```python
from build123d import *

# Parameters (mm, degrees)
CROQUIS1_W              = 91.2
CROQUIS1_H              = 54
SALIENTE_EXTRUIR1_DEPTH = 2
CROQUIS2_R              = 2.5
SALIENTE_EXTRUIR2_DEPTH = 4
CROQUIS3_R              = 1.5
CORTAR_EXTRUIR1_DEPTH   = 4
CROQUIS4_W              = 91.2
CROQUIS4_H              = 54
CROQUIS4_W_2            = 85.2
CROQUIS4_H_2            = 48
SALIENTE_EXTRUIR3_DEPTH = 24
CROQUIS7_W              = 87.2
CROQUIS7_H              = 50
CORTAR_EXTRUIR2_DEPTH   = 14
CROQUIS9_W              = 12
CROQUIS9_H              = 25
CORTAR_EXTRUIR3_DEPTH   = 8


with BuildPart() as part:
    # Croquis1 → Saliente-Extruir1 (new body)
    with BuildSketch(Plane(origin=(0, 0, 0), x_dir=(1, 0, 0), z_dir=(0, 1, 0))):
        with Locations((3, 0)):
            Rectangle(CROQUIS1_W, CROQUIS1_H)
    extrude(amount=SALIENTE_EXTRUIR1_DEPTH)

    # Croquis2 → Saliente-Extruir2 (add)
    with BuildSketch(Plane(origin=(0, 2, 0), x_dir=(1, 0, 0), z_dir=(0, 1, 0))):
        with Locations(Location((-9.6, -19, 0), (0, 0, 90))):
            Circle(CROQUIS2_R)
        with Locations(Location((-9.6, 19, 0), (0, 0, 90))):
            Circle(CROQUIS2_R)
        with Locations(Location((33.4, 19, 0), (0, 0, 90))):
            Circle(CROQUIS2_R)
        with Locations(Location((33.4, -19, 0), (0, 0, 90))):
            Circle(CROQUIS2_R)
    extrude(amount=SALIENTE_EXTRUIR2_DEPTH)

    # Croquis3 → Cortar-Extruir1 (cut)
    with BuildSketch(Plane(origin=(0, 6, 0), x_dir=(1, 0, 0), z_dir=(0, 1, 0))):
        with Locations(Location((-9.6, -19, 0), (0, 0, 270))):
            Circle(CROQUIS3_R)
        with Locations(Location((33.4, -19, 0), (0, 0, 270))):
            Circle(CROQUIS3_R)
        with Locations(Location((33.4, 19, 0), (0, 0, 270))):
            Circle(CROQUIS3_R)
        with Locations(Location((-9.6, 19, 0), (0, 0, 270))):
            Circle(CROQUIS3_R)
    extrude(amount=-CORTAR_EXTRUIR1_DEPTH, mode=Mode.SUBTRACT)

    # Croquis4 → Saliente-Extruir3 (add)
    with BuildSketch(Plane(origin=(0, 2, 0), x_dir=(1, 0, 0), z_dir=(0, 1, 0))):
        with Locations((3, 0)):
            Rectangle(CROQUIS4_W, CROQUIS4_H)
        with Locations((3, 0)):
            Rectangle(CROQUIS4_W_2, CROQUIS4_H_2, mode=Mode.SUBTRACT)
    extrude(amount=SALIENTE_EXTRUIR3_DEPTH)

    # Croquis7 → Cortar-Extruir2 (cut)
    with BuildSketch(Plane(origin=(0, 26, 0), x_dir=(1, 0, 0), z_dir=(0, 1, 0))):
        with Locations((3, 0)):
            Rectangle(CROQUIS7_W, CROQUIS7_H)
    extrude(amount=-CORTAR_EXTRUIR2_DEPTH, mode=Mode.SUBTRACT)

    # Croquis9 → Cortar-Extruir3 (cut)
    with BuildSketch(Plane(origin=(0, 26, 0), x_dir=(1, 0, 0), z_dir=(0, 1, 0))):
        with Locations((-25, -23)):
            Rectangle(CROQUIS9_W, CROQUIS9_H)
    extrude(amount=-CORTAR_EXTRUIR3_DEPTH, mode=Mode.SUBTRACT)


solid = part.part
```
The listing builds one solid part. Answer for the finished solid, in the listing's coordinates (mm). A direction names the side the tool comes from. Give positions to 0.01 mm unless a question says otherwise; leave off trailing zeros. Order: outer loops, then holes, each group sorted by start corner. A loop starts at its lowest first (then second) coordinate and runs counter-clockwise, first axis right, second up. Notation, with made-up numbers: M 24.5,53 L 52.5,53 A26 cw 52.5,70 Z; hole C 76,4.5 d6. An arc over 180 degrees is marked long. Put each result on its own line as item: value. Start each with the question number.
Item 1: Find the intervals of material crossed by line 1 along X through (y, z) = (3.45, 19); line 2 along X through (y, z) = (2.5, -17); line 3 along X through (y, z) = (10.75, 20.5), in increasing order.
Item 2: The part is cut by section C-C, the plane z = -19. Determine the outline of the cut face in (x, y).
Item 3: Which of the six approach directions +Z, -Z, +X, -X, +Y, -Y give full straight-line access (tool end or side, diameter ignored) to faces 1 (the face through (2, 13, -27)), 2 (the face through (32.5, 4, -20.2)), 3 (the face through (-25, 18, 26))?
Item 4: The part is cut by section B-B, the plane x = -24. Determine the outline of the cut face in (y, z).
Item 5: The part is cut by section D-D, the plane y = 19.5. Determine the outline of the cut face in (x, z), and give its area (3 significant figures).
Item 6: The part is cut by section A-A, the plane y = 9.5. Determine the outline of the cut face in (x, z), and give its area (3 significant figures).
Item 7: For a pull along Z with two mould halves and no side action, classify faces 4 (the face through (2, 0, 0)), 5 (the face through (2, 13, 27)), 6 (the face through (-9.53, 4.03, -20.5)) as +Z half, -Z half, draft (parallel to the pull), parting line (faces both ways), or undercut.
Item 8: Flat-ended cylindrical pins translate along their axes: P1, Ø2.5, axis at x = 34.5, z = 18, coming from the +Y side; P2, Ø0.9, axis at x = 33.5, z = 19.5, coming from the +Y side; P3, Ø1.6, axis at x = -27, z = 25.5, coming from the +Y side. Find the tip coordinate at first contact, or state that the pin passes through.
Answer key:
1. line 1: x = -42.6 to -39.6, -12.1 to -11.1, -8.1 to -7.1, 30.9 to 31.9, 34.9 to 35.9, 45.6 to 48.6
1. line 2: x = -42.6 to -39.6, -11.1 to -8.1, 31.9 to 34.9, 45.6 to 48.6
1. line 3: x = -42.6 to -39.6, 45.6 to 48.6
2. outline: M -42.6,0 L 48.6,0 L 48.6,26 L 46.6,26 L 46.6,12 L 45.6,12 L 45.6,2 L 35.9,2 L 35.9,6 L 34.9,6 L 34.9,2 L 31.9,2 L 31.9,6 L 30.9,6 L 30.9,2 L -7.1,2 L -7.1,6 L -8.1,6 L -8.1,2 L -11.1,2 L -11.1,6 L -12.1,6 L -12.1,2 L -39.6,2 L -39.6,12 L -40.6,12 L -40.6,26 L -42.6,26 Z
3. face 1: -Z, +X, -X, +Y, -Y
3. face 2: +Y
3. face 3: +Z, +Y
4. outline: M 0,-27 L 26,-27 L 26,-25 L 12,-25 L 12,-24 L 2,-24 L 2,24 L 12,24 L 12,25 L 18,25 L 18,27 L 0,27 Z
5. outline: M -42.6,-27 L 48.6,-27 L 48.6,27 L -19,27 L -19,25 L 46.6,25 L 46.6,-25 L -40.6,-25 L -40.6,25 L -31,25 L -31,27 L -42.6,27 Z
5. area: 541 mm²
6. outline: M -42.6,-27 L 48.6,-27 L 48.6,27 L -42.6,27 Z; hole M -39.6,-24 L 45.6,-24 L 45.6,24 L -39.6,24 Z
6. area: 835 mm²
7. face 4: draft
7. face 5: +Z half
7. face 6: undercut
8. P1: stops at y = 6
8. P2: stops at y = 2
8. P3: stops at y = 18
